Could you check a few things on this drawing? It's one solid part, dimensions in mm from its lowest x, y, z. A direction names the side the tool comes from. Coordinates: 2 decimals unless noted, no trailing zeros. Write each loop counter-clockwise with the first axis right and the second up, starting at its lowest first coordinate (ties: lowest second). Pieces come first, ordered by that corner, then holes. Notation, with made-up numbers: M 70,6 L 120,6 A8 cw 120,15 Z; hole C -23,-23.5 d8. An arc over 180 degrees is marked long. Use a Markdown table: item, result.
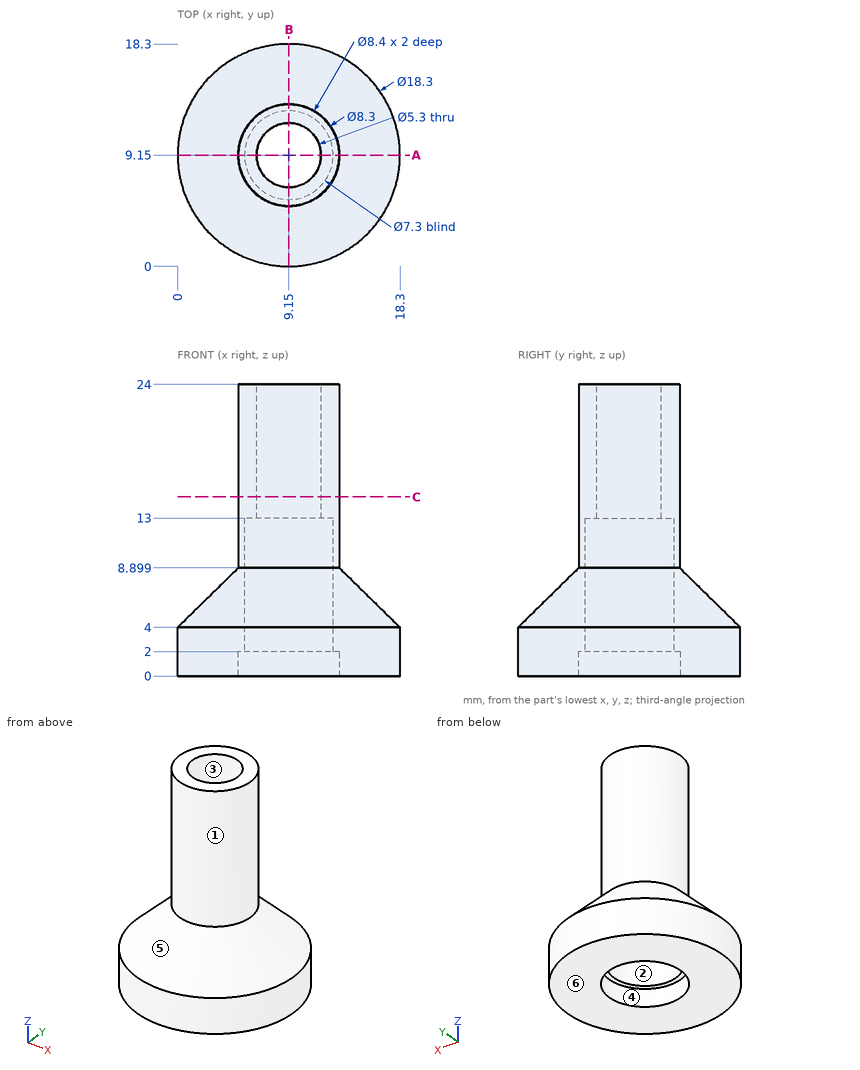
1. Will these pins go through, and if not, where does the flat tip stop? pin 1 Ø3 at (x, z) = (10, 14.5) entering from -Y; pin 2 Ø6 at (y, z) = (11.5, 19) entering from +X; pin 3 Ø3 at (x, y) = (9.15, 9.15) entering from -Z; pin 4 Ø5 at (y, z) = (15, 4) entering from -X.
Answers follow:
| item | result |
|---|---|
| pin 1 | stops at y = 5 |
| pin 2 | stops at x = 13.3 |
| pin 3 | passes through |
| pin 4 | stops at x = 0.64 |
2. Suppose I cut it at A-A on y = 9.15. Write out the boundary of the cut face in (x, z), and give its area (3 significant figures).
Answers follow:
| item | result |
|---|---|
| outline | M 0,0 L 4.95,0 L 4.95,2 L 5.5,2 L 5.5,13 L 6.5,13 L 6.5,24 L 5,24 L 5,8.9 L 0,4 Z; M 11.8,13 L 12.8,13 L 12.8,2 L 13.35,2 L 13.35,0 L 18.3,0 L 18.3,4 L 13.3,8.9 L 13.3,24 L 11.8,24 Z |
| area | 108 mm2 |
3. We'd pull the mould along X, two halves only. Please class the marked faces 4, 5 and 6: +X half, -X half, draft (parallel to the pull), parting line (faces both ways), or undercut.
Answers follow:
| item | result |
|---|---|
| face 4 | undercut |
| face 5 | parting line |
| face 6 | draft |
4. Suppose I cut it at C-C on z = 14.75. Write out the boundary of the cut face in (x, y), and give its area (3 significant figures).
Answers follow:
| item | result |
|---|---|
| outline | C 9.15,9.15 d8.3; hole C 9.15,9.15 d5.3 |
| area | 32.0 mm2 |
5. I need wall thicknesses on probe 1 along X at (y, z) = (9.15, 19.5); probe 2 along Y at (x, z) = (9.15, 1.05); probe 3 along X at (y, z) = (8, 19). Which ranges of each line are inside material? Lowest first, please.
Answers follow:
| item | result |
|---|---|
| probe 1 | x = 5 to 6.5, 11.8 to 13.3 |
| probe 2 | y = 0 to 4.95, 13.35 to 18.3 |
| probe 3 | x = 5.16 to 6.76, 11.54 to 13.14 |
6. Which directions (+Z, -Z, +X, -X, +Y, -Y) give clear straight access to the entire face, cutting with the end or side of a thin tool? Please do the marked faces 1, 2 and 3.
Answers follow:
| item | result |
|---|---|
| face 1 | +Z |
| face 2 | -Z |
| face 3 | +Z, -Z |
